Here's how the part is built. I have some questions about the finished solid (model axes, mm). A direction names the side the tool comes from. Coordinates: 2 decimals unless noted, no trailing zeros. Order: outer loops, then holes, each group sorted by start corner. A loop starts at its lowest first (then second) coordinate and runs counter-clockwise, first axis right, second up. Notation, with made-up numbers: (-40, 83) - (3, 83) arc R34 ccw to (3, 120) - close; hole circle Ø2 at (60.5, 34.5). An arc over 180 degrees is marked (long way). Use one line per item in the form item = value. Start each with the question number.
from build123d import *

# Parameters (mm, degrees)
PAD016_DEPTH    = 46.1772
SKETCH026_W     = 20.32
SKETCH026_H     = 10.16
POCKET004_DEPTH = 2.9972
FILLET_R        = 2.54


with BuildPart() as part:
    # Sketch019 → Pad016 (new body)
    with BuildSketch(Plane.XY.offset(-33.9852)):
        with BuildLine():
            Line((-60.96, 46.1772), (60.96, 46.1772))
            ThreePointArc((76.6572, 30.48), (72.059597, 41.579597), (60.96, 46.1772))
            Line((76.6572, 30.48), (76.6572, -30.48))
            ThreePointArc((60.96, -46.1772), (72.059597, -41.579597), (76.6572, -30.48))
            Line((60.96, -46.1772), (-60.96, -46.1772))
            ThreePointArc((-76.6572, -30.48), (-72.059597, -41.579597), (-60.96, -46.1772))
            Line((-76.6572, -30.48), (-76.6572, 30.48))
            ThreePointArc((-60.96, 46.1772), (-72.059597, 41.579597), (-76.6572, 30.48))
        make_face()
        with BuildLine():
            Line((-60.96, 43.18), (60.96, 43.18))
            ThreePointArc((73.66, 30.48), (69.940256, 39.460256), (60.96, 43.18))
            Line((73.66, 30.48), (73.66, -30.48))
            ThreePointArc((60.96, -43.18), (69.940256, -39.460256), (73.66, -30.48))
            Line((60.96, -43.18), (-60.96, -43.18))
            ThreePointArc((-73.66, -30.48), (-69.940256, -39.460256), (-60.96, -43.18))
            Line((-73.66, -30.48), (-73.66, 30.48))
            ThreePointArc((-60.96, 43.18), (-69.940256, 39.460256), (-73.66, 30.48))
        make_face(mode=Mode.SUBTRACT)
    extrude(amount=-PAD016_DEPTH)

    # Sketch026 → Pocket004 (cut)
    with BuildSketch(Plane(origin=(0, 46.1772, -33.9852), x_dir=(-1, 0, 0), z_dir=(0, 1, 0))):
        with Locations((38.1, -35.56)):
            Rectangle(SKETCH026_W, SKETCH026_H)
    extrude(amount=-POCKET004_DEPTH, mode=Mode.SUBTRACT)

    # Fillet
    fillet_edges = [part.edges().sort_by_distance(p)[0] for p in [
        (-27.94, 44.6786, -64.4652),
        (-27.94, 44.6786, -74.6252),
        (-48.26, 44.6786, -74.6252),
        (-48.26, 44.6786, -64.4652),
    ]]
    fillet(fillet_edges, radius=FILLET_R)


solid = part.part
1) Which directions (+Z, -Z, +X, -X, +Y, -Y) give clear straight access to the entire face, cutting with the end or side of a thin tool? Please do faces 4 (the flat face through (-73.66, 0, -57)), 5 (the cylindrical face through (72.18, 41.46, -56.75)), 6 (the flat face through (-48.26, 45, -70)).
2) If we mould it in two halves opening along Y, with no side actions, what happens to faces 1 (the cylindrical face through (-71.94, 41.7, -56.75)), 2 (the flat face through (1, -43.18, -57)), 3 (the flat face through (17, -44, -33.985))? For each: pulls with the +Y half, pulls with the -Y half, needs draft (parallel to the pull), parting line crosses it, or undercut.
3) I need wall thicknesses on probe 1 along X at (y, z) = (19, -71); probe 2 along Y at (x, z) = (-45, -62.5); probe 3 along X at (y, z) = (-42, -69.5). Which ranges of each line are inside material? Lowest first, please. Write a range as [from, to].
4) Suppose I cut it at D-D, the plane x = -37. List the corners of the cut face in (y, z) for me.
5) For pin 1 (1.5 mm diameter, centred on y = 36.5, z = -39, fed in from +X); pin 2 (0.9 mm diameter, centred on y = 44, z = -69, fed in from +X); pin 3 (3.5 mm diameter, centred on y = 44, z = -70.5, fed in from -X), each with a flat end and sliding along its axis, tell me the tip position at first contact or that it passes through.
6) Suppose I cut it at C-C, the plane z = -54. List the corners of the cut face in (x, y) for me, then the cut area to 3 significant figures.
7) Suppose I cut it at A-A, the plane x = 1.5. List the corners of the cut face in (y, z) for me, then the cut area to 3 significant figures.
8) Suppose I cut it at B-B, the plane y = -8. List the corners of the cut face in (x, z) for me, then the cut area to 3 significant figures.
From the geometry:
q1.face_4 = +Z, -Z
q1.face_5 = +Z, -Z, +X, +Y
q1.face_6 = +Y
q2.face_1 = pulls with the +Y half
q2.face_2 = undercut
q2.face_3 = needs draft
q3.probe_1 = [-76.66, -73.66], [73.66, 76.66]
q3.probe_2 = [-46.18, -43.18], [43.18, 46.18]
q3.probe_3 = [-71.62, -66.31], [66.31, 71.62]
q4.outline = (-46.18, -80.16) - (-43.18, -80.16) - (-43.18, -33.99) - (-46.18, -33.99) - close; (43.18, -80.16) - (46.18, -80.16) - (46.18, -74.63) - (43.18, -74.63) - close; (43.18, -64.47) - (46.18, -64.47) - (46.18, -33.99) - (43.18, -33.99) - close
q5.pin_1 = 75.75
q5.pin_2 = 69.65
q5.pin_3 = -71.35
q6.outline = (-76.66, -30.48) arc R15.7 ccw to (-60.96, -46.18) - (60.96, -46.18) arc R15.7 ccw to (76.66, -30.48) - (76.66, 30.48) arc R15.7 ccw to (60.96, 46.18) - (-60.96, 46.18) arc R15.7 ccw to (-76.66, 30.48) - close; hole (-73.66, -30.48) arc R12.7 ccw to (-60.96, -43.18) - (60.96, -43.18) arc R12.7 ccw to (73.66, -30.48) - (73.66, 30.48) arc R12.7 ccw to (60.96, 43.18) - (-60.96, 43.18) arc R12.7 ccw to (-73.66, 30.48) - close
q6.area = 1,360 mm2
q7.outline = (-46.18, -80.16) - (-43.18, -80.16) - (-43.18, -33.99) - (-46.18, -33.99) - close; (43.18, -80.16) - (46.18, -80.16) - (46.18, -33.99) - (43.18, -33.99) - close
q7.area = 277 mm2
q8.outline = (-76.66, -80.16) - (-73.66, -80.16) - (-73.66, -33.99) - (-76.66, -33.99) - close; (73.66, -80.16) - (76.66, -80.16) - (76.66, -33.99) - (73.66, -33.99) - close
q8.area = 277 mm2
